Geometry: see drawing. Coordinates: mm, zero at the bounding-box minimum. Round coordinates to 2 decimals unless told otherwise and drop trailing zeros. Write each loop counter-clockwise with the first axis right and the second up, starting at its lowest first coordinate (ties: lowest second). Pieces come first, ordered by that corner, then holes.
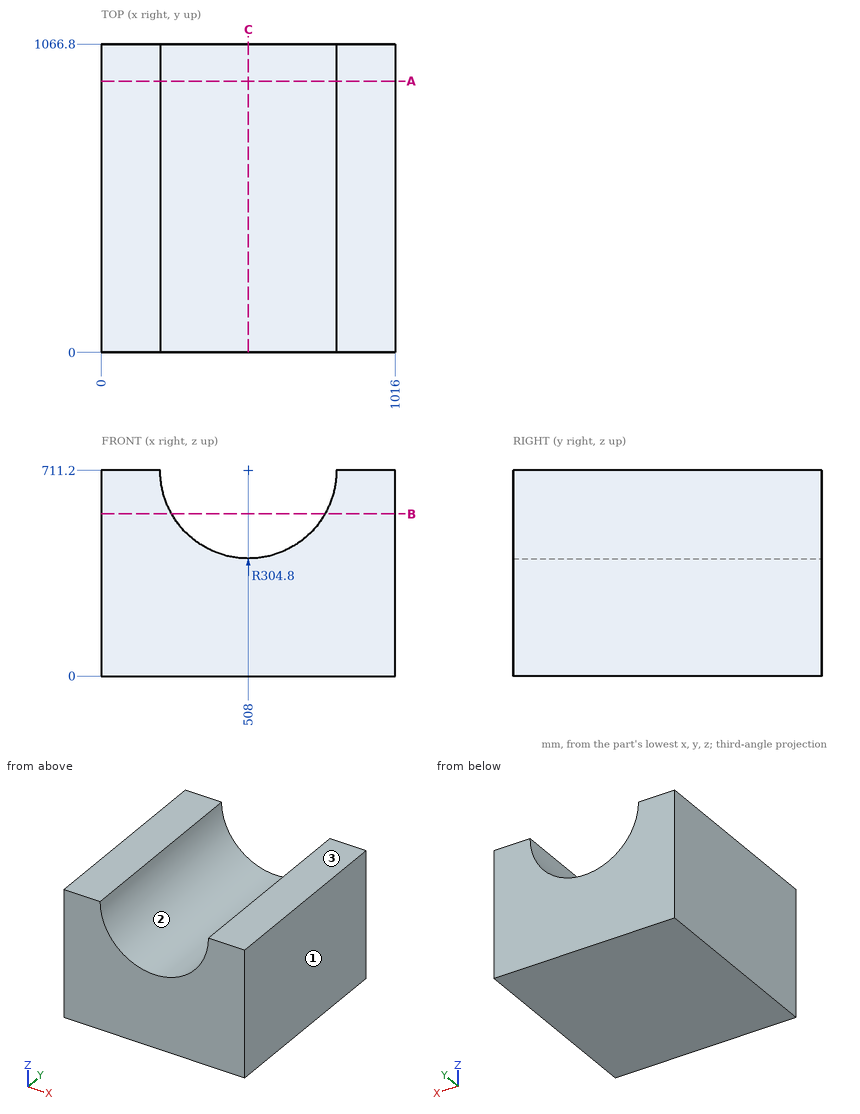
1) Pull-direction query (X, two-part tool) for the marked faces 1, 2 and 3; classes: released by +X, released by -X, zero draft, split by the parting line, or undercut.
Taken from the geometry:
face 1: released by +X
face 2: undercut
face 3: zero draft
2) Section query A-A on y = 938.5. Return the cut outline in (x, z).
Taken from the geometry:
outline: (0, 0) - (1016, 0) - (1016, 711.2) - (812.8, 711.2) arc R304.8 cw to (203.2, 711.2) - (0, 711.2) - close
3) Section query C-C on x = 508. Return the cut outline in (y, z), then the cut area to 3 significant figures.
Taken from the geometry:
outline: (0, 0) - (1066.8, 0) - (1066.8, 406.4) - (0, 406.4) - close
area: 434,000 mm2
4) Material intervals for line 1 (X direction, y = 299, z = 566.5); line 2 (X direction, y = 84.5, z = 629); line 3 (Z direction, x = 446, y = 337), sorted ascending.
Taken from the geometry:
line 1: x = 0 to 239.74, 776.26 to 1016
line 2: x = 0 to 214.49, 801.51 to 1016
line 3: z = 0 to 412.77
5) Section query B-B on z = 560.5. Return the cut outline in (x, y).
Taken from the geometry:
outline: (0, 0) - (243.06, 0) - (243.06, 1066.8) - (0, 1066.8) - close; (772.94, 0) - (1016, 0) - (1016, 1066.8) - (772.94, 1066.8) - close
6) Contact query for flat-ended pins moving along their axis: P1, Ø10, axis at x = 520, y = 373, coming from the +Z side; P2, Ø2, axis at x = 703, y = 815.5, coming from the +Z side. Output: stop coordinate, or through.
Taken from the geometry:
P1: stops at z = 406.87
P2: stops at z = 477.78
